Source: three-view drawing plus pictorial views. Frame: mm from the lowest corner of the part. Coordinates: 2 decimals unless noted, no trailing zeros. Write each loop counter-clockwise with the first axis right and the second up, starting at its lowest first coordinate (ties: lowest second). Pieces come first, ordered by that corner, then holes. Notation, with made-up numbers: (64.25, -6.75) -> (72.25, -6.75) arc R31 cw to (72.25, 24.25) -> close; hole circle Ø3 at (35.5, 59.5). An arc over 180 degrees is marked (long way). Write item = value, one per line.
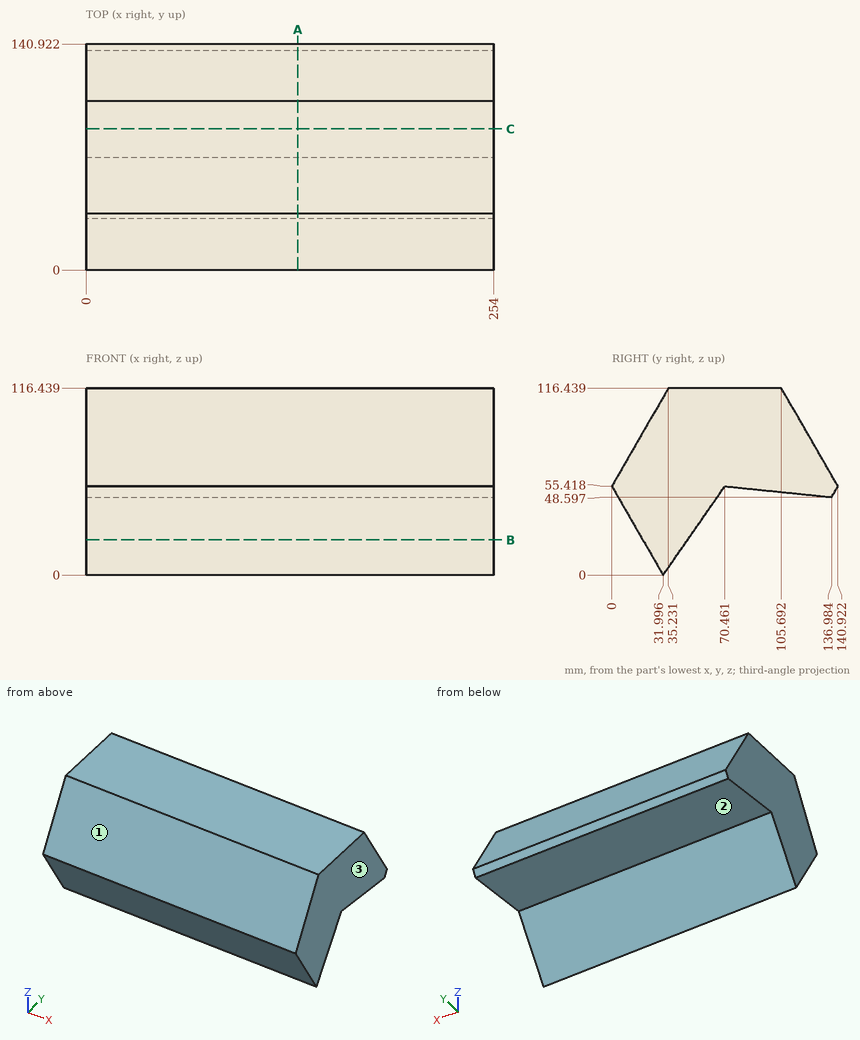
1) Cut plane B-B, the plane z = 22. Output: boundary loops of the cut face in (x, y) (1 decimal).
Answer block:
outline = (0, 19.3) -> (254, 19.3) -> (254, 47.3) -> (0, 47.3) -> close
2) Cut plane A-A, the plane x = 132. Output: boundary loops of the cut face in (y, z) (1 decimal), and give its area (3 significant figures).
Answer block:
outline = (0, 55.4) -> (32, 0) -> (70.5, 55.4) -> (137, 48.6) -> (140.9, 55.4) -> (105.7, 116.4) -> (35.2, 116.4) -> close
area = 8,640 mm2
3) Material intervals for probe 1 along Y at (x, z) = (60, 97) (1 decimal); probe 2 along Y at (x, z) = (135, 105) (1 decimal); probe 3 along Z at (x, y) = (16, 20) (1 decimal), sorted ascending. Write a range as [from, to].
Answer block:
probe_1 = [24, 116.9]
probe_2 = [28.6, 112.3]
probe_3 = [20.8, 90.1]
4) First-contact query: pin 1 Ø8 at (y, z) = (69.5, 56.5) entering from -X; pin 2 Ø8 at (x, y) = (61.5, 82) entering from -Z (1 decimal); pin 3 Ø5 at (x, z) = (134.5, 24) entering from -Y (1 decimal); pin 4 Ø8 at (x, z) = (197.5, 83.5) entering from +Y. Flat tips, straight axial feed; report the tip coordinate or a pass-through.
Answer block:
pin_1 = 0
pin_2 = 53.8
pin_3 = 16.7
pin_4 = 127.02
5) Pull-direction query (Y, two-part tool) for the marked faces 1, 2 and 3; classes: +Y half, -Y half, draft (parallel to the pull), parting line (faces both ways), or undercut.
Answer block:
face_1 = -Y half
face_2 = undercut
face_3 = draft
6) Cut plane C-C, the plane y = 88. Output: boundary loops of the cut face in (x, z).
Answer block:
outline = (0, 53.62) -> (254, 53.62) -> (254, 116.44) -> (0, 116.44) -> close
